Design review of the part built by this model. Coordinates are the model's own, in mm. A direction names the side the tool comes from. Give positions to 0.01 mm unless a question says otherwise; leave off trailing zeros. Order: outer loops, then holes, each group sorted by start corner. A loop starts at its lowest first (then second) coordinate and runs counter-clockwise, first axis right, second up. Notation, with made-up numbers: M 39,71.25 L 43,71.25 A20 cw 43,83.25 Z; hole C 11.5,-14 d7. An arc over 180 degrees is marked long. Answer as a JSON object with one key per item and string values.
from build123d import *

# Parameters (mm, degrees)
BOSS_EXTRU_1_DEPTH = 6


with BuildPart() as part:
    # Esquisse1 → Boss.-Extru.1 (new body)
    with BuildSketch(Plane.XY):
        with BuildLine():
            Line((-16.024411517, 60.322401795), (0, 145.75))
            Line((0, 145.75), (20, 124.149355617))
            Line((20, 124.149355617), (18.328771536, 60.506183401))
            ThreePointArc((18.328771536, 60.506183401), (21.130165565, 55.883417087), (26.499081063, 56.509933866))
            Line((26.499081063, 56.509933866), (93.686294112, 111.650977585))
            Line((93.686294112, 111.650977585), (95.122556403, 82.248171793))
            Line((95.122556403, 82.248171793), (52.933278584, 34.568918325))
            ThreePointArc((52.933278584, 34.568918325), (52.107814004, 29.226972506), (56.62335911, 26.255839844))
            Line((56.62335911, 26.255839844), (143.535730002, 25.309221895))
            Line((143.535730002, 25.309221895), (125.736211496, 1.862154301))
            Line((125.736211496, 1.862154301), (62.769716295, -7.543527827))
            ThreePointArc((62.769716295, -7.543527827), (58.703637157, -11.105097332), (60.25293813, -16.283653443))
            Line((60.25293813, -16.283653443), (126.223202602, -72.875))
            Line((126.223202602, -72.875), (97.516495827, -79.395185884))
            Line((97.516495827, -79.395185884), (43.235506143, -46.126273471))
            ThreePointArc((43.235506143, -46.126273471), (37.831376065, -46.240968709), (35.689497763, -51.203844311))
            Line((35.689497763, -51.203844311), (49.84943589, -136.96019948))
            Line((49.84943589, -136.96019948), (23.667727986, -123.502636215))
            Line((23.667727986, -123.502636215), (3.470922159, -63.126023122))
            ThreePointArc((3.470922159, -63.126023122), (-0.742606336, -59.740176916), (-5.573455253, -62.165187359))
            Line((-5.573455253, -62.165187359), (-49.84943589, -136.96019948))
            Line((-49.84943589, -136.96019948), (-61.255432817, -109.821830482))
            Line((-61.255432817, -109.821830482), (-37.917744879, -50.588404986))
            ThreePointArc((-37.917744879, -50.588404986), (-38.969114979, -45.286292406), (-44.228526613, -44.038748352))
            Line((-44.228526613, -44.038748352), (-126.223202602, -72.875))
            Line((-126.223202602, -72.875), (-117.516495827, -44.754169733))
            Line((-117.516495827, -44.754169733), (-61.564277679, -14.37990993))
            ThreePointArc((-61.564277679, -14.37990993), (-58.961541631, -9.642448378), (-62.188578826, -5.306089555))
            Line((-62.188578826, -5.306089555), (-143.535730002, 25.309221895))
            Line((-143.535730002, 25.309221895), (-118.790284389, 41.254464422))
            Line((-118.790284389, 41.254464422), (-56.404200742, 28.557104797))
            ThreePointArc((-56.404200742, 28.557104797), (-51.365207668, 30.51320441), (-51.049903857, 35.909347515))
            Line((-51.049903857, 35.909347515), (-93.686294112, 111.650977585))
            Line((-93.686294112, 111.650977585), (-64.480778678, 107.959676181))
            Line((-64.480778678, 107.959676181), (-24.851971415, 58.131932813))
            ThreePointArc((-24.851971415, 58.131932813), (-19.734522177, 56.391389738), (-16.024411517, 60.322401795))
        make_face()
        with BuildLine():
            Line((-7.5, 10.310795314), (-7.5, -10.310795314))
            ThreePointArc((-7.5, -10.310795314), (0, -12.75), (7.5, -10.310795314))
            Line((7.5, -10.310795314), (7.5, 10.310795314))
            ThreePointArc((7.5, 10.310795314), (0, 12.75), (-7.5, 10.310795314))
        make_face(mode=Mode.SUBTRACT)
    extrude(amount=BOSS_EXTRU_1_DEPTH)


solid = part.part
(1) To check wall thickness, follow L1, parallel to X at y = 105.5, z = 1.6; L2, parallel to Y at x = -69, z = 4.7; L3, parallel to Y at x = -76, z = 1.3. State the ranges of each line that lie inside material, in increasing order. Write a range as from..to.
Checked values:
{"L1": "x = -90.22..-62.52, -7.55..19.51, 86.19..93.99", "L2": "y = -52.75..-18.42, -2.74..31.12, 67.8..108.53", "L3": "y = -55.21..-22.22, -0.11..32.55, 80.23..109.42"}
(2) Draft analysis for pull direction Y (two halves, no side actions). For faces 1 (the flat face through (-72.07, 73.25, 2.96)), 2 (the flat face through (112.07, -76.09, 2.96)), 3 (the flat face through (9.86, 135.1, 2.96)), state which applies: +Y half, -Y half, draft (parallel to the pull), parting line (faces both ways), or undercut.
Checked values:
{"face 1": "undercut", "face 2": "-Y half", "face 3": "+Y half"}
(3) Tool access review of faces 4 (the flat face through (-10, 5, 6)), 5 (the flat face through (-84.652, -58.255, 2.958)), 6 (the flat face through (-44.94, 83.39, 2.96)), 7 (the flat face through (-121.93, -59.01, 2.96)), 8 (the flat face through (74.32, 58.74, 2.96)): name each direction out of +Z, -Z, +X, -X, +Y, -Y from which nothing blocks a thin tool from reaching the whole face with its end or side.
Checked values:
{"face 4": "+Z, +X, -X, +Y, -Y", "face 5": "+Z, -Z", "face 6": "+Z, -Z, +Y", "face 7": "+Z, -Z, -X", "face 8": "+Z, -Z, +X"}
(4) We need section A-A (x = -74.5). Write out the cut boundary in (y, z), plus the area to 3 significant figures.
Checked values:
{"outline": "M -54.68,0 L -21.4,0 L -21.4,6 L -54.68,6 Z; M -0.67,0 L 32.24,0 L 32.24,6 L -0.67,6 Z; M 77.57,0 L 109.23,0 L 109.23,6 L 77.57,6 Z", "area": "587 mm^2"}
(5) We need section C-C (x = -21). Write out the cut boundary in (y, z).
Checked values:
{"outline": "M -88.23,0 L 56.24,0 L 56.24,6 L -88.23,6 Z"}
(6) We need section B-B (x = 73). Write out the cut boundary in (y, z).
Checked values:
{"outline": "M -64.37,0 L -27.22,0 L -27.22,6 L -64.37,6 Z; M -6.02,0 L 26.08,0 L 26.08,6 L -6.02,6 Z; M 57.25,0 L 94.67,0 L 94.67,6 L 57.25,6 Z"}
(7) Insertion check: pin 1 (1.5 mm diameter, centred on y = 91.5, z = 3, fed in from -X); pin 2 (2 mm diameter, centred on y = 21.5, z = 3, fed in from +X); pin 3 (1.5 mm diameter, centred on x = 39, z = 2, fed in from -Y). Each pin has a flat end and moves straight along its axis. Give the tip position at first contact, or say it passes through.
Checked values:
{"pin 1": "stops at x = -82.77", "pin 2": "stops at x = 141.4", "pin 3": "stops at y = -131.77"}
